from build123d import *

# Parameters (mm, degrees)
F0_W     = 74.814543128
F0_H     = 71.3509097695
F1_DEPTH = 12.7
F3_DEPTH = 38.1
F4_DEPTH = 38.1
F6_DEPTH = 6.35
F6_TAPER = -3


with BuildPart() as f1:
    # F0 (on Top) → F1 (new body)
    with BuildSketch(Plane.XY):
        Rectangle(F0_W, F0_H)
    extrude(amount=F1_DEPTH)

    # F2 (on face) → F3 (join)
    with BuildSketch(Plane(origin=(0, 0, 0), x_dir=(1, 0, 0), z_dir=(0, 0, -1))):
        with BuildLine():
            Line((27.0553643694, -35.6754548848), (37.407271564, -35.6754548848))
            ThreePointArc((37.407271564, -35.6754548848), (0, -8.418886875), (-37.407271564, -35.6754548848))
            Line((-37.407271564, -35.6754548848), (-27.0553643694, -35.6754548848))
            ThreePointArc((-27.0553643694, -35.6754548848), (0, -18.1025332163), (27.0553643694, -35.6754548848))
        make_face()
        with BuildLine():
            ThreePointArc((-37.407271564, -35.6754548848), (-6.0941405685, -86.5382776277), (39.2973991584, -47.7162860334))
            ThreePointArc((39.2973991584, -47.7162860334), (38.8219915943, -41.6221454649), (37.407271564, -35.6754548848))
            Line((37.407271564, -35.6754548848), (27.0553643694, -35.6754548848))
            ThreePointArc((27.0553643694, -35.6754548848), (28.9670953732, -41.5614715317), (29.6137528171, -47.7162860334))
            ThreePointArc((29.6137528171, -47.7162860334), (-6.1548145016, -76.6833814066), (-27.0553643694, -35.6754548848))
            Line((-27.0553643694, -35.6754548848), (-37.407271564, -35.6754548848))
        make_face()
    extrude(amount=-F3_DEPTH)

    # F4 (cut, symmetric): a face of the model
    f4_faces = [f1.faces().sort_by_distance(p)[0] for p in [
        (0, 28.4298339612, 12.7),
    ]]
    extrude(f4_faces, amount=F4_DEPTH, both=True, mode=Mode.SUBTRACT)

    # F5 (on Right) → F6 (join, symmetric)
    with BuildSketch(Plane.YZ):
        Polygon((-16.0677041858, 12.7), (8.418886875, 12.7), (8.418886875, 35.9063632786), align=None)
    extrude(amount=F6_DEPTH, both=True, taper=F6_TAPER)


solid = f1.part
Verification items for the finished model (mm, model axes). A direction names the side the tool comes from. Coordinates: 2 decimals unless noted, no trailing zeros. Loops run counter-clockwise (first coordinate to the right, second up) from the corner with the lowest first, then second, coordinate; pieces in that order, holes last. Notation, with made-up numbers: M 51,65 L 95,65 A16 cw 95,87 Z; hole C -40,89.5 d3. An arc over 180 degrees is marked long. One line per item, written item: value.
1. Section check C-C on x = -17.5. Record the cut outline in (y, z).
Answers follow:
outline: M -35.68,0 L 23.83,0 L 23.83,38.1 L 12.53,38.1 L 12.53,12.7 L -35.68,12.7 Z; M 71.61,0 L 82.9,0 L 82.9,38.1 L 71.61,38.1 Z
2. Section check D-D on y = 38.5. Record the cut outline in (x, z).
Answers follow:
outline: M -38.2,0 L -28.14,0 L -28.14,38.1 L -38.2,38.1 Z; M 28.14,0 L 38.2,0 L 38.2,38.1 L 28.14,38.1 Z
3. Section check A-A on y = 56. Record the cut outline in (x, z).
Answers follow:
outline: M -38.41,0 L -28.43,0 L -28.43,38.1 L -38.41,38.1 Z; M 28.43,0 L 38.41,0 L 38.41,38.1 L 28.43,38.1 Z
4. Gauge pin test, flat ends, axial feed: P1, Ø6, axis at x = -29, z = 19, coming from the +Y side; P2, Ø12, axis at x = 18.5, y = -12.5, coming from the -Z side; P3, Ø12, axis at y = 25, z = 7, coming from the -X side; P4, Ø6.5, axis at y = 6.5, z = 9, coming from the +X side. Record the tip position at first contact, or that the pin passes through.
Answers follow:
P1: y = 77.18
P2: z = 0
P3: x = -37.41
P4: x = 37.41
5. Section check B-B on x = 24.5. Record the cut outline in (y, z).
Answers follow:
outline: M -35.68,0 L 31.08,0 L 31.08,38.1 L 16.99,38.1 L 16.99,12.7 L -35.68,12.7 Z; M 64.35,0 L 78.44,0 L 78.44,38.1 L 64.35,38.1 Z
6. Material ranges on line 1 along Y through (x, z) = (0, 10); line 2 along X through (y, z) = (62.5, 4.5); line 3 along Z through (x, y) = (-35, 7.5), recorded low to high. Write a range as from..to.
Answers follow:
line 1: -35.68..18.1, 77.33..87.01
line 2: -36.41..-25.66, 25.66..36.41
line 3: 0..12.7
7. Mould release check, pull along X, two halves, no side actions. Record for faces 1 (the flat face through (-6.35, -1, 21)), 2 (the flat face through (6.35, -1, 21)), 3 (the cylindrical face through (-6.42, 18.807, 18.783)), 4 (the flat face through (-1, -35.675, 6)): pulls with the +X half, pulls with the -X half, needs draft (parallel to the pull), parting line crosses it, or undercut.
Answers follow:
face 1: pulls with the -X half
face 2: pulls with the +X half
face 3: undercut
face 4: needs draft
8. Set-up check for faces 5 (the flat face through (-1, 13, 0)), 6 (the flat face through (-37.407, 0, 6)), 7 (the flat face through (37.407, 0, 6)): record each of +Z, -Z, +X, -X, +Y, -Y from which the full face is reachable in a straight line by a thin tool's end or side.
Answers follow:
face 5: -Z, +X, -X, +Y, -Y
face 6: +Z, -Z, -X, -Y
face 7: +Z, -Z, +X, -Y
